```python
from build123d import *

# Parameters (mm, degrees)
BOSS_EXTRUDE2_DEPTH = 5
SKETCH3_R           = 2
CUT_EXTRUDE1_DEPTH  = 48.696960071
SKETCH4_R           = 7.5
BOSS_EXTRUDE5_DEPTH = 1
SKETCH6_R           = 5
BOSS_EXTRUDE6_DEPTH = 5


with BuildPart() as part:
    # Sketch1 → Boss-Extrude2 (new body)
    with BuildSketch(Plane.XY):
        with BuildLine():
            Line((-30, 15), (45, 15))
            Line((45, 15), (45, -15))
            Line((45, -15), (-30, -15))
            ThreePointArc((-30, -15), (-45, 0), (-30, 15))
        make_face()
    extrude(amount=BOSS_EXTRUDE2_DEPTH)

    # Sketch3 → Cut-Extrude1 (cut, through all)
    with BuildSketch(Plane(origin=(0, 0, 0), x_dir=(-1, 0, 0), z_dir=(0, 0, -1))):
        with Locations((-40, 0)):
            Circle(SKETCH3_R)
        with Locations((-25, 0)):
            Circle(SKETCH3_R)
    extrude(amount=-CUT_EXTRUDE1_DEPTH, mode=Mode.SUBTRACT)

    # Sketch4 → Boss-Extrude5 (add)
    with BuildSketch(Plane(origin=(0, 0, 0), x_dir=(-1, 0, 0), z_dir=(0, 0, -1))):
        with Locations(Location((20, 0, 0), (0, 0, 180))):
            Circle(SKETCH4_R)
    extrude(amount=BOSS_EXTRUDE5_DEPTH)

    # Sketch6 → Boss-Extrude6 (add)
    with BuildSketch(Plane(origin=(0, 0, -1), x_dir=(-1, 0, 0), z_dir=(0, 0, -1))):
        with Locations((20, 0)):
            Circle(SKETCH6_R)
    extrude(amount=BOSS_EXTRUDE6_DEPTH)


solid = part.part
```
The listing builds one solid part. Answer for the finished solid, in the listing's coordinates (mm). A direction names the side the tool comes from. Round coordinates to 2 decimals unless told otherwise and drop trailing zeros. Loops run counter-clockwise (first coordinate to the right, second up) from the corner with the lowest first, then second, coordinate; pieces in that order, holes last. Notation, with made-up numbers: (-3, 82) - (34, 82) arc R22 ccw to (34, 115) - close; hole circle Ø2 at (74, 44.5). An arc over 180 degrees is marked (long way). Return JSON: item names as keys, results as strings. Group by question number.
1. The part is cut by section B-B on y = 0. Determine the outline of the cut face in (x, z).
2. Which of the six approach directions +Z, -Z, +X, -X, +Y, -Y give full straight-line access (tool end or side, diameter ignored) to faces 1 (the flat face through (7, 15, 2)), 2 (the flat face through (-18, 5, -1))?
3. Each of these flat-tipped pins is pushed along its axis until it touches: P1, Ø3, axis at y = -11.5, z = 0, coming from the -X side; P2, Ø3, axis at y = 5.5, z = -3.5, coming from the +X side; P3, Ø3.5, axis at x = 40, y = 0, coming from the +Z side; P4, Ø1, axis at x = 25.5, y = -1.5, coming from the -Z side. Where does it stop, or does it pass through?
4. The mould has two halves that part along Y. Classify faces 3 (the flat face through (45, 0, 2)), 4 (the cylindrical face through (42, 0, 2)), 5 (the cylindrical face through (-15, 0, -3)): pulls with the +Y half, pulls with the -Y half, needs draft (parallel to the pull), parting line crosses it, or undercut.
5. The part is cut by section A-A on x = 25. Determine the outline of the cut face in (y, z), then the cut area to 3 significant figures.
6. Consider probe 1 along Y at (x, z) = (25, 2.6); probe 2 along Z at (x, y) = (39, -4.5); probe 3 along X at (y, z) = (4.25, 1.25). Determine where each line is inside the solid, lowest interval first.
7. The part is cut by section C-C on x = -20. Determine the outline of the cut face in (y, z).
8. The part is cut by section D-D on y = 6. Determine the outline of the cut face in (x, z), then the cut area to 3 significant figures.
Resolved:
{
 "1": {"outline": "(-45, 0) - (-27.5, 0) - (-27.5, -1) - (-25, -1) - (-25, -6) - (-15, -6) - (-15, -1) - (-12.5, -1) - (-12.5, 0) - (23, 0) - (23, 5) - (-45, 5) - close; (27, 0) - (38, 0) - (38, 5) - (27, 5) - close; (42, 0) - (45, 0) - (45, 5) - (42, 5) - close"},
 "2": {"face 1": "+Z, -Z, +X, -X, +Y", "face 2": "-Z"},
 "3": {"P1": "stops at x = -41.18", "P2": "stops at x = -17", "P3": "passes through", "P4": "stops at z = 0"},
 "4": {"face 3": "needs draft", "face 4": "undercut", "face 5": "parting line crosses it"},
 "5": {"outline": "(-15, 0) - (-2, 0) - (-2, 5) - (-15, 5) - close; (2, 0) - (15, 0) - (15, 5) - (2, 5) - close", "area": "130 mm²"},
 "6": {"probe 1": "y = -15 to -2, 2 to 15", "probe 2": "z = 0 to 5", "probe 3": "x = -44.39 to 45"},
 "7": {"outline": "(-15, 0) - (-7.5, 0) - (-7.5, -1) - (-5, -1) - (-5, -6) - (5, -6) - (5, -1) - (7.5, -1) - (7.5, 0) - (15, 0) - (15, 5) - (-15, 5) - close"},
 "8": {"outline": "(-43.75, 0) - (-24.5, 0) - (-24.5, -1) - (-15.5, -1) - (-15.5, 0) - (45, 0) - (45, 5) - (-43.75, 5) - close", "area": "453 mm²"}
}
